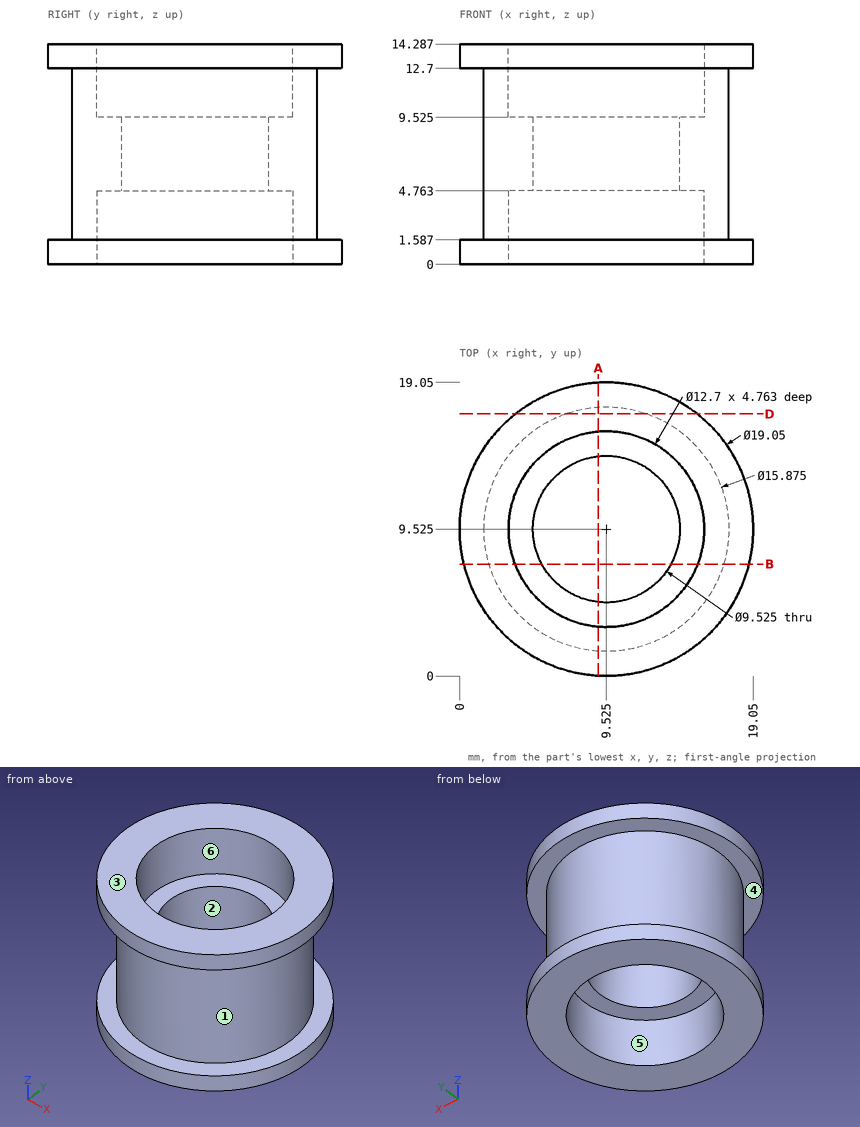
Verification items for this drawing (mm, ordinates from the low corner). A direction names the side the tool comes from. Round coordinates to 2 decimals unless told otherwise and drop trailing zeros. Loops run counter-clockwise (first coordinate to the right, second up) from the corner with the lowest first, then second, coordinate; pieces in that order, holes last. Notation, with made-up numbers: M -20.75,14 L -8.75,14 A22 cw -8.75,26 Z; hole C 84,-17 d6. An arc over 180 degrees is marked long. Answer as a JSON object with one key per item and string values.
1. Section check A-A (x = 9). Record the boundary of the cut face in (y, z) (1 decimal).
Reply:
{"outline": "M 0,0 L 3.2,0 L 3.2,4.8 L 4.8,4.8 L 4.8,9.5 L 3.2,9.5 L 3.2,14.3 L 0,14.3 L 0,12.7 L 1.6,12.7 L 1.6,1.6 L 0,1.6 Z; M 14.3,4.8 L 15.9,4.8 L 15.9,0 L 19,0 L 19,1.6 L 17.4,1.6 L 17.4,12.7 L 19,12.7 L 19,14.3 L 15.9,14.3 L 15.9,9.5 L 14.3,9.5 Z"}
2. Gauge pin test, flat ends, axial feed: P1, Ø8, axis at x = 14.5, y = 9, coming from the +Z side; P2, Ø4, axis at x = 10.5, y = 10, coming from the +Z side; P3, Ø3, axis at y = 3.5, z = 6.5, coming from the +X side (1 decimal); P4, Ø3, axis at x = 5, z = 5, coming from the +Y side. Record the tip position at first contact, or that the pin passes through.
Reply:
{"P1": "stops at z = 14.29", "P2": "passes through", "P3": "stops at x = 16", "P4": "stops at y = 16.86"}
3. Section check D-D (y = 17). Record the boundary of the cut face in (x, z) (1 decimal).
Reply:
{"outline": "M 3.6,0 L 15.4,0 L 15.4,1.6 L 12.2,1.6 L 12.2,12.7 L 15.4,12.7 L 15.4,14.3 L 3.6,14.3 L 3.6,12.7 L 6.9,12.7 L 6.9,1.6 L 3.6,1.6 Z"}
4. Scan lines: line 1 (Z direction, x = 4.5, y = 15.75); line 2 (X direction, y = 6.75, z = 9.25) (1 decimal); line 3 (X direction, y = 12, z = 1). Record each from-to range of solid material in increasing order.
Reply:
{"line 1": "z = 0 to 1.59, 12.7 to 14.29", "line 2": "x = 2.1 to 5.7, 13.4 to 17", "line 3": "x = 0.33 to 3.68, 15.37 to 18.72"}
5. Mould release check, pull along X, two halves, no side actions. Record for the marked faces 1, 2 and 3: pulls with the +X half, pulls with the -X half, needs draft (parallel to the pull), parting line crosses it, or undercut.
Reply:
{"face 1": "parting line crosses it", "face 2": "undercut", "face 3": "needs draft"}
6. Access from +Z, -Z, +X, -X, +Y, -Y to the whole of each face (thin tool, end or side, straight path). Record for the marked faces 4, 5 and 6.
Reply:
{"face 4": "none", "face 5": "-Z", "face 6": "+Z"}
7. Section check B-B (y = 7.25). Record the boundary of the cut face in (x, z) (1 decimal).
Reply:
{"outline": "M 0.3,0 L 3.6,0 L 3.6,4.8 L 5.3,4.8 L 5.3,9.5 L 3.6,9.5 L 3.6,14.3 L 0.3,14.3 L 0.3,12.7 L 1.9,12.7 L 1.9,1.6 L 0.3,1.6 Z; M 13.7,4.8 L 15.5,4.8 L 15.5,0 L 18.8,0 L 18.8,1.6 L 17.1,1.6 L 17.1,12.7 L 18.8,12.7 L 18.8,14.3 L 15.5,14.3 L 15.5,9.5 L 13.7,9.5 Z"}
